Can you work these out from the model? Positions are in its coordinate system, mm. A direction names the side the tool comes from. Coordinates: 2 decimals unless noted, no trailing zeros. Write each loop counter-clockwise with the first axis right and the second up, starting at its lowest first coordinate (ties: lowest second). Pieces come first, ordered by that corner, then holes. Notation, with made-up numbers: (6.25, 37) -> (49.25, 37) arc R25 cw to (49.25, 58) -> close; hole circle Ø11 at (21.5, 67). An arc over 180 degrees is marked (long way). Use one line per item in the form item = value.
```python
from build123d import *

# Parameters (mm, degrees)
SKETCH1_R           = 1.75
SKETCH1_R_2         = 2.4
BOSS_EXTRUDE1_DEPTH = 5
EXTRUDE_START       = 3
SKETCH_1_R          = 4
SKETCH_1_R_2        = 1.75
EXTRUDE_1_DEPTH     = 3


with BuildPart() as part:
    # Sketch1 → Boss-Extrude1 (new body)
    with BuildSketch(Plane(origin=(0, 4, 0), x_dir=(1, 0, 0), z_dir=(0, 1, 0))):
        with BuildLine():
            Line((1.43808022, 3.600125745), (2.081641936, 4))
            ThreePointArc((2.081641936, 4), (2.861028333, 4.588201733), (3.521749436, 5.30713988))
            ThreePointArc((3.521749436, 5.30713988), (3.405395609, 5.596745198), (3.282888305, 5.883801663))
            ThreePointArc((3.282888305, 5.883801663), (1.93527598, 5.894040025), (0.627094961, 5.57027124))
            ThreePointArc((0.627094961, 5.57027124), (0.366286148, 6.046375), (0.084372603, 6.510293938))
            ThreePointArc((0.084372603, 6.510293938), (1.018855105, 7.48132754), (1.683794586, 8.65351323))
            ThreePointArc((1.683794586, 8.65351323), (1.496450048, 8.903135899), (1.303821399, 9.148703928))
            ThreePointArc((1.303821399, 9.148703928), (-0.000522033, 8.809805691), (-1.180330337, 8.158486898))
            ThreePointArc((-1.180330337, 8.158486898), (-1.555477026, 8.550865528), (-1.947855656, 8.926012217))
            ThreePointArc((-1.947855656, 8.926012217), (-1.296536862, 10.105820521), (-0.957638625, 11.410163953))
            ThreePointArc((-0.957638625, 11.410163953), (-1.203206655, 11.602792602), (-1.452829324, 11.79013714))
            ThreePointArc((-1.452829324, 11.79013714), (-2.625015014, 11.125197659), (-3.596048616, 10.190715157))
            ThreePointArc((-3.596048616, 10.190715157), (-4.059967554, 10.472628702), (-4.536071314, 10.733437515))
            ThreePointArc((-4.536071314, 10.733437515), (-4.212302529, 12.041618533), (-4.222540891, 13.389230859))
            ThreePointArc((-4.222540891, 13.389230859), (-4.509597355, 13.511738163), (-4.799202674, 13.62809199))
            ThreePointArc((-4.799202674, 13.62809199), (-5.759348103, 12.682425791), (-6.455432668, 11.528463019))
            ThreePointArc((-6.455432668, 11.528463019), (-6.976508546, 11.680699536), (-7.503891752, 11.809396783))
            ThreePointArc((-7.503891752, 11.809396783), (-7.529737283, 13.156800143), (-7.888414517, 14.455843809))
            ThreePointArc((-7.888414517, 14.455843809), (-8.197396993, 14.499881098), (-8.507248835, 14.537314892))
            ThreePointArc((-8.507248835, 14.537314892), (-9.18992168, 13.375367565), (-9.563620196, 12.080565177))
            ThreePointArc((-9.563620196, 12.080565177), (-10.106342554, 12.09275), (-10.649064912, 12.080565177))
            ThreePointArc((-10.649064912, 12.080565177), (-11.022763428, 13.375367565), (-11.705436272, 14.537314892))
            ThreePointArc((-11.705436272, 14.537314892), (-12.015288115, 14.499881098), (-12.324270591, 14.455843809))
            ThreePointArc((-12.324270591, 14.455843809), (-12.682947825, 13.156800143), (-12.708793355, 11.809396783))
            ThreePointArc((-12.708793355, 11.809396783), (-13.236176561, 11.680699536), (-13.757252439, 11.528463019))
            ThreePointArc((-13.757252439, 11.528463019), (-14.453337005, 12.682425791), (-15.413482434, 13.62809199))
            ThreePointArc((-15.413482434, 13.62809199), (-15.703087752, 13.511738163), (-15.990144217, 13.389230859))
            ThreePointArc((-15.990144217, 13.389230859), (-16.000382579, 12.041618533), (-15.676613793, 10.733437515))
            ThreePointArc((-15.676613793, 10.733437515), (-16.152717554, 10.472628702), (-16.616636492, 10.190715157))
            ThreePointArc((-16.616636492, 10.190715157), (-17.587670094, 11.125197659), (-18.759855783, 11.79013714))
            ThreePointArc((-18.759855783, 11.79013714), (-19.009478453, 11.602792602), (-19.255046482, 11.410163953))
            ThreePointArc((-19.255046482, 11.410163953), (-18.916148245, 10.105820521), (-18.264829452, 8.926012217))
            ThreePointArc((-18.264829452, 8.926012217), (-18.657208082, 8.550865528), (-19.032354771, 8.158486898))
            ThreePointArc((-19.032354771, 8.158486898), (-20.212163074, 8.809805691), (-21.516506507, 9.148703928))
            ThreePointArc((-21.516506507, 9.148703928), (-21.709135156, 8.903135899), (-21.896479694, 8.65351323))
            ThreePointArc((-21.896479694, 8.65351323), (-21.231540213, 7.48132754), (-20.297057711, 6.510293938))
            ThreePointArc((-20.297057711, 6.510293938), (-20.578971255, 6.046375), (-20.839780068, 5.57027124))
            ThreePointArc((-20.839780068, 5.57027124), (-22.147961087, 5.894040025), (-23.495573413, 5.883801663))
            ThreePointArc((-23.495573413, 5.883801663), (-23.618080717, 5.596745198), (-23.734434544, 5.30713988))
            ThreePointArc((-23.734434544, 5.30713988), (-22.788768345, 4.346994451), (-21.634805572, 3.650909885))
            ThreePointArc((-21.634805572, 3.650909885), (-21.803584999, 3.067429176), (-21.942853375, 2.47620963))
            Line((-21.942853375, 2.47620963), (-41.11537681, -0.047900965))
            ThreePointArc((-41.11537681, -0.047900965), (-44.559051487, -4.53578518), (-40.071167272, -7.979459856))
            Line((-40.071167272, -7.979459856), (-20.898643838, -5.455349261))
            ThreePointArc((-20.898643838, -5.455349261), (-7.038913378, -11.697242445), (1.974222624, 0.542722358))
            ThreePointArc((1.974222624, 0.542722358), (3.269025011, 0.916420874), (4.430972339, 1.599093719))
            ThreePointArc((4.430972339, 1.599093719), (4.393538544, 1.908945561), (4.349501255, 2.217928037))
            ThreePointArc((4.349501255, 2.217928037), (3.050457589, 2.576605271), (1.70305423, 2.602450802))
            ThreePointArc((1.70305423, 2.602450802), (1.581217534, 3.104116905), (1.43808022, 3.600125745))
        make_face()
        with Locations(Location((-40.593272041, -4.013680411, 0), (0, 0, 90))):
            Circle(SKETCH1_R, mode=Mode.SUBTRACT)
        with Locations(Location((-10.106342554, 0, 0), (0, 0, 90))):
            Circle(SKETCH1_R_2, mode=Mode.SUBTRACT)
    extrude(amount=-BOSS_EXTRUDE1_DEPTH)

    # 草图1 → 凸台-拉伸1 (add)
    with BuildSketch(Plane(origin=(0, 4, 0), x_dir=(1, 0, 0), z_dir=(0, 1, 0)).offset(EXTRUDE_START)):
        with Locations(Location((-40.593272041, -4.013680411, 0), (0, 0, 270))):
            Circle(SKETCH_1_R)
        with Locations(Location((-40.593272041, -4.013680411, 0), (0, 0, 270))):
            Circle(SKETCH_1_R_2, mode=Mode.SUBTRACT)
    extrude(amount=-EXTRUDE_1_DEPTH)


solid = part.part
```
Q1. Suppose I cut it at B-B (y = 6). Write out the boundary of the cut face in (x, z).
Return value:
outline = circle Ø8 at (-40.59, 4.01); hole circle Ø3.5 at (-40.59, 4.01)
Q2. Will these pins go through, and if not, where does the flat tip stop? pin 1 (5 mm diameter, centred on x = -33, z = 9, fed in from +Y); pin 2 (1.5 mm diameter, centred on x = -23, y = 5.5, fed in from -Z); pin 3 (1 mm diameter, centred on y = 2.5, z = 5.5, fed in from +X); pin 4 (4 mm diameter, centred on y = 4.5, z = 9, fed in from -X).
Return value:
pin_1 = 4
pin_2 = through
pin_3 = 0.9
pin_4 = -43.25
Q3. Suppose I cut it at C-C (z = 9.75). Write out the boundary of the cut face in (x, y).
Return value:
outline = (-17.26, -1) -> (-2.95, -1) -> (-2.95, 4) -> (-17.26, 4) -> close
Q4. For faces 4 (the cylindrical face through (-9.182, 1.535, -13.393)), 5 (the cylindrical face through (-16.146, 1.535, -10.476)), which set-ups out of +Z, -Z, +X, -X, +Y, -Y let a thin tool reach every point of the face, with its end or its side?
Return value:
face_4 = -Z, +Y, -Y
face_5 = +Y, -Y
Q5. Suppose I cut it at A-A (z = 3.5). Write out the boundary of the cut face in (x, y).
Return value:
outline = (-44.56, -1) -> (-42.27, -1) -> (-42.27, 7) -> (-44.56, 7) -> close; (-38.92, -1) -> (1.47, -1) -> (1.47, 4) -> (-36.63, 4) -> (-36.63, 7) -> (-38.92, 7) -> close
Q6. If I drill on line 1 (Y direction, x = -1.5, z = -5); line 2 (Z direction, x = -40, y = 1.75); line 3 (X direction, y = 4.5, z = 4.25), over which ranges is the centre line in solid material (lowest first)? Write a range as from..to.
Return value:
line_1 = -1..4
line_2 = -0.1..2.37, 5.66..7.97
line_3 = -44.59..-42.33, -38.86..-36.6
Q7. Thinking about a two-plate mould opening in X: for faces 1 (the cylindrical face through (-20.19, 1.54, -8.8)), 2 (the cylindrical face through (2.85, 1.54, -4.58)), 3 (the cylindrical face through (-21.8, 1.54, -3.08)), which applies, released by +X, released by -X, zero draft, split by the parting line, or undercut?
Return value:
face_1 = undercut
face_2 = released by +X
face_3 = released by -X
Q8. Suppose I cut it at D-D (y = 0.5). Give the number of separate pieces and of enclosed holes in the cut face, then the cut area to 3 significant figures.
Return value:
separate_pieces = 1
enclosed_holes = 2
area = 652 mm2
